Autodesk Inventor part; units mm, degrees
ref_plane "Work Plane1" through (12.7, 12.7, 25.4) normal (1, 0, 0) x (0, 0, -1)
ref_plane "YZ Plane" through (0, 0, 0) normal (1, 0, 0) x (0, 1, 0)
ref_plane "XZ Plane" through (0, 0, 0) normal (0, 1, 0) x (-1, 0, 0)
sketch "Sketch1" plane through (0, 0, 0) normal (0, 0, 1) x (1, 0, 0)
  line L0 (0, 0) -> (25.4, 0)
  line L1 (25.4, 0) -> (25.4, 25.4)
  line L2 (25.4, 25.4) -> (0, 25.4)
  line L3 (0, 25.4) -> (0, 0)
  dimension "d0" = 25.4
  dimension "d1" = 25.4
extrude "Extrusion1" add sketch "Sketch1" along normal blind 25.4
sketch "Sketch2" plane through (0, 25.4, 0) normal (0, 1, 0) x (1, 0, 0)
  line L0 (0, 0) -> (0, -25.4)
  line L1 (25.4, -25.4) -> (0, -25.4)
  circle A0 centre (12.7, -12.7) radius 6.35
  dimension "d4" = 12.7
  dimension "d5" = 12.7
  dimension "d6" = 12.7
sketch "Sketch3" plane through (0, 0, 25.4) normal (0, 0, 1) x (1, 0, 0)
  line L0 (25.4, 25.4) -> (0, 25.4)
  line L1 (0, 25.4) -> (0, 0)
  circle A0 centre (12.7, 12.7) radius 6.35
  dimension "d7" = 12.7
  dimension "d8" = 12.7
  dimension "d9" = 12.7
sketch "Sketch4" plane through (0, 0, 0) normal (0, -1, 0) x (1, 0, 0)
  line L0 (25.4, 0) -> (25.4, 25.4)
  line L1 (0, 25.4) -> (25.4, 25.4)
  circle A0 centre (12.7, 12.7) radius 6.35
  point P0 (0, 0)
  dimension "d10" = 12.7
  dimension "d11" = 12.7
  dimension "d12" = 12.7
sketch "Sketch5" plane through (0, 0, 0) normal (0, 0, -1) x (-1, 0, 0)
  line L0 (-25.4, 0) -> (-25.4, 25.4)
  line L1 (0, 0) -> (-25.4, 0)
  circle A0 centre (-12.7, 12.7) radius 6.35
  dimension "d13" = 12.7
  dimension "d14" = 12.7
  dimension "d15" = 12.7
ref_plane "Work Plane1" through (12.7, 12.7, 25.4) normal (1, 0, 0) x (0, 0, -1)
sketch "Sketch6" plane through (12.7, 12.7, 25.4) normal (1, 0, 0) x (0, 0, -1)
  line L0 (25.4, -12.7) -> (25.4, 12.7)
  arc A0 (25.4, 0) -> (12.7731, 12.6779) centre (7.1702, -5.5295) ccw
  arc A1 (25.4, 0) -> (12.7731, 12.6779) centre (25.4731, 12.6998) ccw
  arc A2 (0, 0) -> (12.3568, -13.1392) centre (-6.0452, -18.0654) ccw
  dimension "d17" = 19.05
  dimension "d18" = 12.7
  dimension "d19" = 19.05
sweep "Sweep1" add profiles "Sketch3" path "Sketch6" path curves A2
sketch "Sketch7" plane through (12.7, 12.7, 25.4) normal (1, 0, 0) x (0, 0, -1)
  arc A0 (25.3272, -0.0369) -> (12.0094, 12.137) centre (24.6991, 12.6475) ccw
  point P0 (25.4, -12.7)
  dimension "d23" = 12.7
sweep "Sweep2" add profiles "Sketch5" path "Sketch7"
fillet "Fillet1" radius 3.175 1 edges at (25.4, 25.4, 12.7)
fillet "Fillet2" radius 3.175 3 edges at (24.4701, 24.4701, 0) (11.1125, 25.4, 0) (25.4, 11.1125, 0)
fillet "Fillet3" radius 3.175 3 edges at (24.4701, 24.4701, 25.4) (11.1125, 25.4, 25.4) (25.4, 11.1125, 25.4)
fillet "Fillet4" radius 3.175 5 edges at (24.4701, 0, 24.4701) (11.1125, 0, 25.4) (24.4701, 0, 0.9299) (11.1125, 0, 0) (25.4, 0, 12.7)
fillet "Fillet5" radius 3.175 8 edges at (0, 0.9299, 24.4701) (0, 12.7, 25.4) (0, 24.4701, 24.4701) (0, 25.4, 12.7) (0, 24.4701, 0.9299) (0, 12.7, 0) (0, 0.9299, 0.9299) (0, 0, 12.7)
properties part number "Lauren's funky piece"
Could you check a few things on this model? Use its own coordinates, in mm. A direction names the side the tool comes from. Round coordinates to 2 decimals unless told otherwise and drop trailing zeros. Order: outer loops, then holes, each group sorted by start corner. A loop starts at its lowest first (then second) coordinate and runs counter-clockwise, first axis right, second up.
(1) If we mould it in two halves opening along Y, with no side actions, what happens to faces 4 (the cylindrical face through (12.83, 24.49, 24.45)), 5 (the flat face through (13, 0, 13)), 6 (the cylindrical face through (0.91, 12.57, 0.95))? For each: released by +Y, released by -Y, zero draft, split by the parting line, or undercut.
Response values:
face 4: released by +Y
face 5: undercut
face 6: zero draft
(2) Imagine slicing it at B-B (x = 8.5). Count the separate pieces of the cut face and the enclosed holes in it, plus the area to 3 significant figures.
Response values:
separate pieces: 1
enclosed holes: 2
area: 2,100 mm2
(3) Please list where these lines run through material, in increasing order: line 1 along Z through (x, y) = (7.5, 7); line 2 along Y through (x, z) = (7.75, 3); line 3 along Y through (x, z) = (9, 40).
Response values:
line 1: z = 0 to 25.4, 41.02 to 50.29
line 2: y = 0 to 25.4, 33.74 to 41.83
line 3: y = -27.79 to -16.76, 6.03 to 17.06
(4) Imagine slicing it at A-A (x = 2.25). Write out the boundary of the cut face in (y, z) (3 decimals).
Response values:
outline: (0.138, 3.175) arc R3.037 ccw to (3.175, 0.138) - (22.225, 0.138) arc R3.037 ccw to (25.262, 3.175) - (25.262, 22.225) arc R3.037 ccw to (22.225, 25.262) - (3.175, 25.262) arc R3.037 ccw to (0.138, 22.225) - close
(5) I'm going to push flat-ended pins straight in: pin 1 (12 mm diameter, centred on x = 5, z = 19.5, fed in from +Y); pin 2 (3 mm diameter, centred on x = 8.5, y = -9.5, fed in from +Z); pin 3 (9.5 mm diameter, centred on x = 14, z = 8.5, fed in from +Y). Where does each tip first touch, or does it pass through?
Response values:
pin 1: stops at y = 35.95
pin 2: stops at z = 55.7
pin 3: stops at y = 44.09
(6) Which directions (+Z, -Z, +X, -X, +Y, -Y) give clear straight access to the entire face, cutting with the end or side of a thin tool? Please do faces 1 (the cylindrical face through (0.91, 24.45, 12.57)), 2 (the flat face through (6, 13, 0)), 3 (the cylindrical face through (12.83, 24.45, 0.91)).
Response values:
face 1: +Z, -Z, -X, +Y
face 2: none
face 3: +X, -X
